Source: CAD feature listing. Evaluate the final solid. Frame: model axes, mm. A direction names the side the tool comes from. Give positions to 0.01 mm unless a question says otherwise; leave off trailing zeros. Write each loop counter-clockwise with the first axis right and the second up, starting at its lowest first coordinate (ties: lowest second). Pieces come first, ordered by that corner, then holes. Notation, with made-up numbers: M 82,41.25 L 117,41.25 A30 ccw 117,74.25 Z; hole C 81,64.5 d2. An arc over 180 degrees is marked long. Return JSON: item names as keys, results as strings.
```python
from build123d import *

# Parameters (mm, degrees)
SKETCH1_W           = 60
SKETCH1_H           = 40
BOSS_EXTRUDE1_DEPTH = 30
SKETCH2_OUTSIDE_W   = 57.62
SKETCH2_OUTSIDE_H   = 47.62
SKETCH2_OUTSIDE_W_2 = 40
SKETCH2_OUTSIDE_H_2 = 30
SKETCH2_OUTSIDE_W_3 = 35
SKETCH2_OUTSIDE_H_3 = 25
CUT_EXTRUDE1_DEPTH  = 57.5
SKETCH3_R           = 2.5
CUT_EXTRUDE2_DEPTH  = 57.5
FILLET1_R           = 1
SKETCH4_R           = 5
CUT_EXTRUDE3_DEPTH  = 20


with BuildPart() as part:
    # Sketch1 → Boss-Extrude1 (new body)
    with BuildSketch(Plane(origin=(0, 0, 0), x_dir=(1, 0, 0), z_dir=(0, 1, 0))):
        with Locations((-10.610539169, 2.437108943)):
            Rectangle(SKETCH1_W, SKETCH1_H)
    extrude(amount=BOSS_EXTRUDE1_DEPTH)

    # Sketch2 outside → Cut-Extrude1 (cut)
    # profile 1 of 2: a face of its own
    with BuildSketch(Plane.ZY.offset(40.610539169)):
        with Locations((-2.437, 15)):
            Rectangle(SKETCH2_OUTSIDE_W, SKETCH2_OUTSIDE_H)
        with Locations((-2.437108943, 15)):
            Rectangle(SKETCH2_OUTSIDE_W_2, SKETCH2_OUTSIDE_H_2, mode=Mode.SUBTRACT)
    # profile 2 of 2: a face of its own
    with BuildSketch(Plane.ZY.offset(40.610539169)):
        with Locations((-2.437108943, 15)):
            Rectangle(SKETCH2_OUTSIDE_W_3, SKETCH2_OUTSIDE_H_3)
    extrude(amount=-CUT_EXTRUDE1_DEPTH, mode=Mode.SUBTRACT)

    # Sketch3 → Cut-Extrude2 (cut)
    with BuildSketch(Plane(origin=(0, 30, 0), x_dir=(1, 0, 0), z_dir=(0, 1, 0))):
        with Locations(Location((-26.75468652, 2.437108943, 0), (0, 0, 270))):
            Circle(SKETCH3_R)
    extrude(amount=-CUT_EXTRUDE2_DEPTH, mode=Mode.SUBTRACT)

    # Fillet1
    fillet1_edges = [part.edges().sort_by_distance(p)[0] for p in [
        (-26.75468652, 2.5, -4.937108943),
    ]]
    fillet(fillet1_edges, radius=FILLET1_R)

    # Sketch4 → Cut-Extrude3 (cut)
    with BuildSketch(Plane(origin=(0, 30, 0), x_dir=(1, 0, 0), z_dir=(0, 1, 0))):
        with Locations(Location((-26.75468652, 2.437108943, 0), (0, 0, 270))):
            Circle(SKETCH4_R)
    extrude(amount=-CUT_EXTRUDE3_DEPTH, mode=Mode.SUBTRACT)


solid = part.part
```
1) Set-up query: faces 1 (the face through (-29.195, 0.761, -2.979)), 2 (the face through (-31.19, 28.77, -0.13)), 3 (the face through (-12, 15, -19.937)). Return all of +Z, -Z, +X, -X, +Y, -Y with unobstructed straight access to the full face (end or side cutting, diameter ignored); none if empty.
Numbers:
{"face 1": "+Y, -Y", "face 2": "+Y", "face 3": "-X"}
2) Line query: line 1 (Z direction, x = -28, y = 27); line 2 (Y direction, x = -32, z = -19); line 3 (X direction, y = 10, z = -5.5). Output: solid intervals per line, ascending. Write a range as [from, to].
Numbers:
{"line 1": "z = [-22.44, -19.94], [15.06, 17.56]", "line 2": "y = [0, 2.5], [27.5, 30]", "line 3": "x = [16.89, 19.39]"}
3) Cut plane A-A, the plane y = 11.25. Return the cut outline in (x, z), then the cut area to 4 significant figures.
Numbers:
{"outline": "M -40.61,-22.44 L 19.39,-22.44 L 19.39,17.56 L -40.61,17.56 L -40.61,15.06 L 16.89,15.06 L 16.89,-19.94 L -40.61,-19.94 Z", "area": "387.5 mm²"}
4) Cut plane B-B, the plane z = 4. Return the cut outline in (x, y), then the cut area to 4 significant figures.
Numbers:
{"outline": "M -40.61,0 L 19.39,0 L 19.39,30 L -40.61,30 L -40.61,27.5 L 16.89,27.5 L 16.89,2.5 L -40.61,2.5 Z", "area": "362.5 mm²"}
5) Draft query along Z for faces 4 (the face through (19.389, 15, -2)), 5 (the face through (-11, 15, 17.563)), 6 (the face through (-12, 2.5, -3)), 7 (the face through (-12, 27.5, -3)). Return one class per face: released by +Z, released by -Z, zero draft, split by the parting line, or undercut.
Numbers:
{"face 4": "zero draft", "face 5": "released by +Z", "face 6": "undercut", "face 7": "undercut"}
6) Contact query for flat-ended pins moving along their axis: pin 1 Ø3 at (x, z) = (-4.5, -4) entering from -Y; pin 2 Ø1 at (y, z) = (19, -5.5) entering from -X. Output: stop coordinate, or through.
Numbers:
{"pin 1": "stops at y = 0", "pin 2": "stops at x = 16.89"}
7) Cut plane C-C, the plane x = -11.5. Return the cut outline in (y, z), then the cut area to 3 significant figures.
Numbers:
{"outline": "M 0,-22.44 L 30,-22.44 L 30,17.56 L 0,17.56 Z; hole M 2.5,-19.94 L 27.5,-19.94 L 27.5,15.06 L 2.5,15.06 Z", "area": "325 mm²"}
8) Cut plane D-D, the plane y = 28.25. Return the cut outline in (x, z).
Numbers:
{"outline": "M -40.61,-22.44 L 19.39,-22.44 L 19.39,17.56 L -40.61,17.56 Z; hole C -26.75,-2.44 d10"}
